Build history of the part. All positions in model axes, mm. A direction names the side the tool comes from. Round coordinates to 2 decimals unless told otherwise and drop trailing zeros. Order: outer loops, then holes, each group sorted by start corner. A loop starts at its lowest first (then second) coordinate and runs counter-clockwise, first axis right, second up. Notation, with made-up numbers: (-33.5, 73.25) - (-23.5, 73.25) arc R9 ccw to (-23.5, 88.25) - close; hole circle Ø9 at (31.5, 36.25). An arc over 180 degrees is marked (long way). One line per question, with ' | ' between items. Start each with the question number.
from build123d import *

# Parameters (mm, degrees)
IRON_V40X40X3_1_DEPTH = 260


with BuildPart() as part:
    # Sketch1 → Iron V40X40X3(1) (new body)
    with BuildSketch(Plane(origin=(0, 0, 0), x_dir=(1, 0, 0), z_dir=(0, 1, 0))):
        with BuildLine():
            Line((0, 0), (0, 40))
            ThreePointArc((0, 40), (2.121320344, 39.121320344), (3, 37))
            Line((3, 37), (3, 6.5))
            ThreePointArc((3, 6.5), (4.025126266, 4.025126266), (6.5, 3))
            Line((6.5, 3), (37, 3))
            ThreePointArc((37, 3), (39.121320344, 2.121320344), (40, 0))
            Line((40, 0), (0, 0))
        make_face()
    extrude(amount=IRON_V40X40X3_1_DEPTH)


solid = part.part
Item 1: Slice it at B-B (x = 15). Write the cut outline in (y, z), plus the area to 3 significant figures.
Item 2: Pin check, flat tips, straight feed: pin 1 (1.5 mm diameter, centred on y = 111.5, z = -4.5, fed in from +X); pin 2 (2 mm diameter, centred on y = 78, z = -16.5, fed in from +X); pin 3 (4 mm diameter, centred on x = 18.5, y = 196.5, fed in from -Z). Stop position of each tip, or through.
Item 3: 3-axis set-ups, long thin cutter, end or side, ignore diameter. For faces 1 (the face through (3, 128, -22)), 2 (the face through (0, 128, -20)): which of +Z, -Z, +X, -X, +Y, -Y reach the whole face in a straight line?
Item 4: Pull direction Z, two halves, no side cores. Call faces 3 (the face through (11, 0, -2)), 4 (the face through (20, 128, 0)), 5 (the face through (22, 128, -3)): released by +Z, released by -Z, zero draft, split by the parting line, or undercut.
Item 5: Wall check: line 1 along X through (y, z) = (15, -25.5); line 2 along Z through (x, y) = (13, 188); line 3 along X through (y, z) = (114, -2). Give the ranges that are in metal, low to high. Write a range as [from, to].
Item 6: Slice it at A-A (y = 167). Write the cut outline in (x, z), plus the area to 3 significant figures.
Item 7: Slice it at C-C (z = -24.5). Write the cut outline in (x, y).
A:
1) outline: (0, -3) - (260, -3) - (260, 0) - (0, 0) - close | area: 780 mm^2
2) pin 1: x = 4.33 | pin 2: x = 3 | pin 3: z = -3
3) face 1: -Z, +X, +Y, -Y | face 2: +Z, -Z, -X, +Y, -Y
4) face 3: zero draft | face 4: released by +Z | face 5: released by -Z
5) line 1: [0, 3] | line 2: [-3, 0] | line 3: [0, 39.24]
6) outline: (0, -40) arc R3 ccw to (3, -37) - (3, -6.5) arc R3.5 cw to (6.5, -3) - (37, -3) arc R3 ccw to (40, 0) - (0, 0) - close | area: 230 mm^2
7) outline: (0, 0) - (3, 0) - (3, 260) - (0, 260) - close
